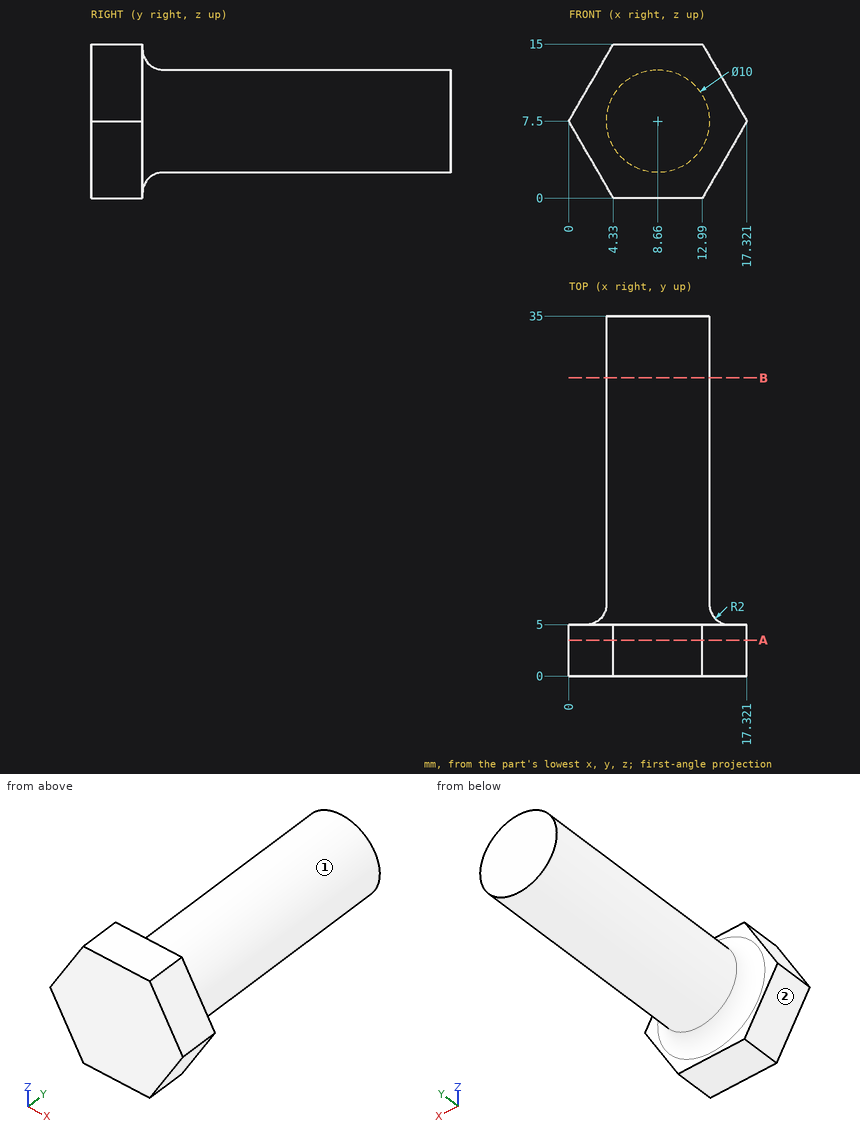
Geometry: see drawing. Coordinates: mm, zero at the bounding-box minimum. A direction names the side the tool comes from. Coordinates: 2 decimals unless noted, no trailing zeros. Loops run counter-clockwise (first coordinate to the right, second up) from the corner with the lowest first, then second, coordinate; pieces in that order, holes last.
(1) Section A-A on y = 3.5. Return the cut outline in (x, z), then the cut area to 3 significant figures.
(2) First-contact query: pin 1 Ø6 at (x, y) = (3, 22) entering from +Z (1 decimal); pin 2 Ø1.5 at (x, z) = (15, 4) entering from +Y (1 decimal); pin 3 Ø6 at (x, y) = (6, 26.5) entering from -Z. Flat tips, straight axial feed; report the tip coordinate or a pass-through.
(3) Material intervals for probe 1 along Y at (x, z) = (1, 8); probe 2 along X at (y, z) = (13, 6.25); probe 3 along Y at (x, z) = (2.5, 9), sorted ascending.
(4) Set-up query: the marked faces 1 and 2. Return all of +Z, -Z, +X, -X, +Y, -Y with unobstructed straight access to the full face (end or side cutting, diameter ignored); none if empty.
(5) Section B-B on y = 29. Return the cut outline in (x, z).
Data:
1. outline: (0, 7.5) - (4.33, 0) - (12.99, 0) - (17.32, 7.5) - (12.99, 15) - (4.33, 15) - close
1. area: 195 mm2
2. pin 1: stops at z = 11.7
2. pin 2: stops at y = 5.1
2. pin 3: stops at z = 2.5
3. probe 1: y = 0 to 5
3. probe 2: x = 3.82 to 13.5
3. probe 3: y = 0 to 5.11
4. face 1: +Y
4. face 2: -Z, -X, +Y, -Y
5. outline: circle Ø10 at (8.66, 7.5)
